Check sheet for the drawn part. Datum: minimum x, y, z corner. Units: mm. Give positions to 0.01 mm unless a question says otherwise; leave off trailing zeros. Loops run counter-clockwise (first coordinate to the right, second up) from the corner with the lowest first, then second, coordinate; pieces in that order, holes last. Notation, with made-up numbers: (79.5, 18) - (97.5, 18) arc R31 cw to (97.5, 47) - close; hole circle Ø6 at (-24.5, 30.25). An arc over 180 degrees is marked (long way). One line per item, written item: value. Start each with the question number.
1. Scan lines: L1, parallel to Y at x = 19.05, z = 1.55; L2, parallel to Y at x = 107.5, z = 0.3; L3, parallel to X at y = 29.5, z = 0.65. Record each from-to range of solid material in increasing order. Write a range as [from, to].
2. Sectioned sample at B-B (x = 19.05). Record the cut outline in (y, z) (1 decimal), plus the area to 3 significant figures.
3. Sectioned sample at A-A (z = 0.85). Record the cut outline in (x, y), plus the area to 3 significant figures.
4. Gauge pin test, flat ends, axial feed: pin 1 (1 mm diameter, centred on x = 83, z = 1.5, fed in from -Y); pin 2 (5 mm diameter, centred on x = 19.05, y = 19.05, fed in from +Z). Record the tip position at first contact, or that the pin passes through.
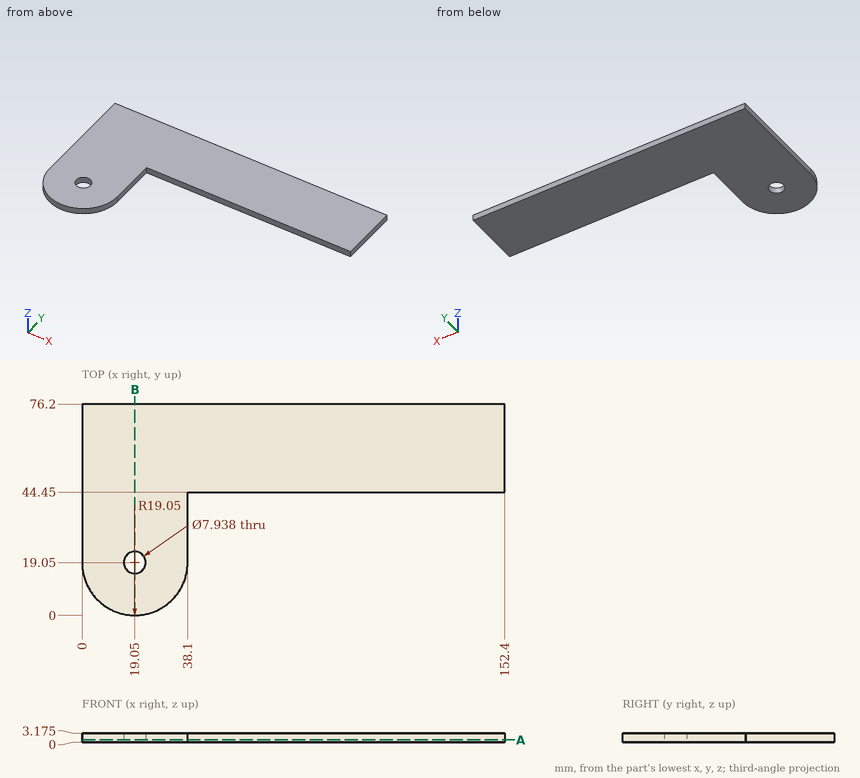
Results are:
1. L1: y = [0, 15.08], [23.02, 76.2]
1. L2: y = [44.45, 76.2]
1. L3: x = [0, 38.1]
2. outline: (0, 0) - (15.1, 0) - (15.1, 3.2) - (0, 3.2) - close; (23, 0) - (76.2, 0) - (76.2, 3.2) - (23, 3.2) - close
2. area: 217 mm^2
3. outline: (0, 19.05) arc R19.05 ccw to (38.1, 19.05) - (38.1, 44.45) - (152.4, 44.45) - (152.4, 76.2) - (0, 76.2) - close; hole circle Ø7.94 at (19.05, 19.05)
3. area: 6,330 mm^2
4. pin 1: stops at y = 44.45
4. pin 2: passes through
